from build123d import *

# Parameters (mm, degrees)
F0_W      = 35
F0_H      = 50
F1_DEPTH  = 3
F2_W      = 18
F2_H      = 13
F2_H_2    = 18
F3_DEPTH  = 24
F4_R      = 7
F5_DEPTH  = 50
F6_R      = 2
F7_DEPTH  = 25
F8_W      = 4
F8_H      = 13
F9_DEPTH  = 10
F10_W     = 4
F10_H     = 13
F11_DEPTH = 10
F12_R     = 1.5
F13_DEPTH = 5
F14_W     = 6
F14_H     = 18
F15_DEPTH = 18


with BuildPart() as f1:
    # F0 (on Front) → F1 (new body)
    with BuildSketch(Plane.XZ):
        with Locations((2.50131, -0.066432)):
            Rectangle(F0_W, F0_H)
    extrude(amount=-F1_DEPTH)

    # F2 (on face) → F3 (join)
    with BuildSketch(Plane(origin=(0, 3, 0), x_dir=(-1, 0, 0), z_dir=(0, 1, 0))):
        with Locations((-2.50131, 18.433568)):
            Rectangle(F2_W, F2_H)
        with Locations((-2.50131, -0.066432)):
            Rectangle(F2_W, F2_H_2)
        with Locations((-2.50131, -18.566432)):
            Rectangle(F2_W, F2_H)
    extrude(amount=F3_DEPTH)

    # F4 (on face) → F5 (cut)
    with BuildSketch(Plane(origin=(0, 0, -25.066432), x_dir=(1, 0, 0), z_dir=(0, 0, -1))):
        with Locations((2.50131, -12)):
            Circle(F4_R)
    extrude(amount=-F5_DEPTH, mode=Mode.SUBTRACT)

    # F6 (on face) → F7 (cut)
    with BuildSketch(Plane(origin=(-6.49869, 0, 0), x_dir=(0, -1, 0), z_dir=(-1, 0, 0))):
        with Locations((-23, 18.433568)):
            Circle(F6_R)
        with Locations((-23, -18.217815)):
            Circle(F6_R)
    extrude(amount=-F7_DEPTH, mode=Mode.SUBTRACT)

    # F8 (on face) → F9 (cut)
    with BuildSketch(Plane(origin=(0, 27, 0), x_dir=(-1, 0, 0), z_dir=(0, 1, 0))):
        with Locations((-2.50131, 18.433568)):
            Rectangle(F8_W, F8_H)
    extrude(amount=-F9_DEPTH, mode=Mode.SUBTRACT)

    # F10 (on face) → F11 (cut)
    with BuildSketch(Plane(origin=(0, 27, 0), x_dir=(-1, 0, 0), z_dir=(0, 1, 0))):
        with Locations((-2.50131, -18.566432)):
            Rectangle(F10_W, F10_H)
    extrude(amount=-F11_DEPTH, mode=Mode.SUBTRACT)

    # F12 (on face) → F13 (cut)
    with BuildSketch(Plane.XZ):
        with Locations((15.50131, 19.933568)):
            Circle(F12_R)
        with Locations((-10.49869, -20.066432)):
            Circle(F12_R)
        with Locations((15.50131, -20.066432)):
            Circle(F12_R)
        with Locations((-10.49869, 19.933568)):
            Circle(F12_R)
    extrude(amount=-F13_DEPTH, mode=Mode.SUBTRACT)

    # F14 (on face) → F15 (cut)
    with BuildSketch(Plane(origin=(-6.49869, 0, 0), x_dir=(0, -1, 0), z_dir=(-1, 0, 0))):
        with Locations((-24, -0.066432)):
            Rectangle(F14_W, F14_H)
    extrude(amount=-F15_DEPTH, mode=Mode.SUBTRACT)


solid = f1.part
Work out the finished part from the listing and answer in its coordinate system (mm). A direction names the side the tool comes from. Give positions to 0.01 mm unless a question says otherwise; leave off trailing zeros. Write each loop counter-clockwise with the first axis right and the second up, starting at its lowest first coordinate (ties: lowest second). Pieces come first, ordered by that corner, then holes. Notation, with made-up numbers: (55.25, 3.5) - (83.25, 3.5) arc R25 cw to (83.25, 35.5) - close; hole circle Ø7 at (27.25, 40). An arc over 180 degrees is marked (long way). One line per item, written item: value. Start each with the question number.
1. For a pull along Z with two mould halves and no side action, classify faces 6 (the flat face through (2, 4, -25.066)), 7 (the flat face through (-14.999, 1, 0)), 8 (the flat face through (2, 21, 0)) as +Z half, -Z half, draft (parallel to the pull), parting line (faces both ways), or undercut.
2. Given pin 1 (1.5 mm diameter, centred on y = 14.5, z = -19.5, fed in from +X); pin 2 (3.5 mm diameter, centred on y = 23, z = 18.43, fed in from +X); pin 3 (9 mm diameter, centred on y = 24, z = 19.5, fed in from -X); pin 4 (1.5 mm diameter, centred on x = 9.5, z = 8, fed in from +Y), each flat-ended and moving along its own axis, determine where each tip first touches the part or whether it passes through.
3. For faces 1 (the flat face through (-6.499, 15, -19)), 2 (the flat face through (0.501, 21, -20)), 3 (the cylindrical face through (14.4, 1.48, -19.05)), 4 (the flat face through (7, 18, -9.066)), 5 (the flat face through (11.501, 15, 18)), determine the directions among +Z, -Z, +X, -X, +Y, -Y from which every point of the face is accessible in a straight line to the end or side of a thin tool.
4. Find section C-C (y = 23). State how many separate pieces and enclosed holes the cut face has, then the cut area to 3 significant figures.
5. Find section A-A (y = 4.25). Write down the section's boundary in (x, z), then the cut area to 3 significant figures.
6. Find section D-D (z = 14.5). Write down the section's boundary in (x, y), then the cut area to 3 significant figures.
7. Consider probe 1 along Z at (x, y) = (-4, 15.25); probe 2 along Z at (x, y) = (-1, 23); probe 3 along X at (y, z) = (12, 1.75). Determine where each line is inside the solid, lowest interval first.
8. Find section B-B (z = -8). Write down the section's boundary in (x, y), then the cut area to 3 significant figures.
Geometry results:
1. face 6: -Z half
1. face 7: draft
1. face 8: undercut
2. pin 1: x = 11.5
2. pin 2: through
2. pin 3: x = -6.5
2. pin 4: y = 21
3. face 1: +Z, -Z, -X, +Y
3. face 2: -Z, +Y
3. face 3: +Y, -Y
3. face 4: +X, -X, +Y
3. face 5: +Z, -Z, +X, +Y
4. separate pieces: 8
4. enclosed holes: 0
4. area: 252 mm2
5. outline: (-6.5, -25.07) - (11.5, -25.07) - (11.5, -12.07) - (-6.5, -12.07) - close; (-6.5, -9.07) - (11.5, -9.07) - (11.5, 8.93) - (-6.5, 8.93) - close; (-6.5, 11.93) - (11.5, 11.93) - (11.5, 24.93) - (-6.5, 24.93) - close
5. area: 792 mm2
6. outline: (-15, 0) - (20, 0) - (20, 3) - (11.5, 3) - (11.5, 27) - (4.5, 27) - (4.5, 18.71) arc R7 cw (long way) to (0.5, 18.71) - (0.5, 27) - (-6.5, 27) - (-6.5, 3) - (-15, 3) - close
6. area: 351 mm2
7. probe 1: -25.07 to -12.07, -9.07 to 8.93, 11.93 to 24.93
7. probe 2: -25.07 to -20.22, -16.22 to -12.07, 11.93 to 16.43, 20.43 to 24.93
7. probe 3: -6.5 to -4.5, 9.5 to 11.5
8. outline: (-15, 0) - (20, 0) - (20, 3) - (11.5, 3) - (11.5, 21) - (-6.5, 21) - (-6.5, 3) - (-15, 3) - close; hole circle Ø14 at (2.5, 12)
8. area: 275 mm2
